Can you work these out from the model? Positions are in its coordinate system, mm. Face numbers are marked on the shaded views. Round coordinates to 2 decimals unless told otherwise and drop trailing zeros. Order: outer loops, then holes, each group sorted by start corner. A loop starts at its lowest first (then second) coordinate and runs counter-clockwise, first axis right, second up. Notation, with made-up numbers: M -38.75,31.25 L -34.75,31.25 A22 ccw -34.75,53.25 Z; hole C -12.5,59 d4. An arc over 180 degrees is marked long. Answer as a JSON object with one key per item and string values. Group by question number.
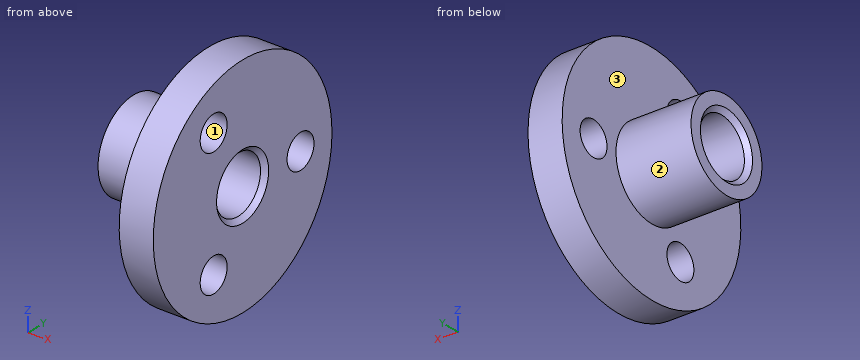
```python
from build123d import *

# Parameters (mm, degrees)
SKETCH_1_R               = 9.95
SKETCH_1_R_2             = 1.5
EXTRUDE_1_DEPTH          = 3
SKETCH_2_R               = 3.95
EXTRUDE_2_DEPTH          = 6.6
CUT_EXTRUDE_1_DEPTH      = 18.034230244
CUT_EXTRUDE_1_DEPTH_BACK = 18.034230244
SKETCH_3_R               = 2.5
CHAMFER_1_SIZE           = 0.4


with BuildPart() as part:
    # Эскиз1 → Бобышка-Вытянуть1 (new body)
    with BuildSketch(Plane(origin=(0, 0, 0), x_dir=(0, 0, -1), z_dir=(1, 0, 0))):
        Circle(SKETCH_1_R)
        with Locations((0, 6.45)):
            Circle(SKETCH_1_R_2, mode=Mode.SUBTRACT)
        with Locations((5.585863854, -3.225)):
            Circle(SKETCH_1_R_2, mode=Mode.SUBTRACT)
        with Locations((-5.585863854, -3.225)):
            Circle(SKETCH_1_R_2, mode=Mode.SUBTRACT)
    extrude(amount=EXTRUDE_1_DEPTH)

    # Эскиз2 → Бобышка-Вытянуть2 (add)
    with BuildSketch(Plane.ZY):
        with Locations(Location((0, 0, 0), (0, 0, 180))):
            Circle(SKETCH_2_R)
    extrude(amount=EXTRUDE_2_DEPTH)

    # Эскиз3 → Вырез-Вытянуть1 (cut, two sides: drawn at the far end of the back side and taken through both)
    with BuildSketch(Plane.ZY.offset(6.6).offset(-CUT_EXTRUDE_1_DEPTH_BACK)):
        Circle(SKETCH_3_R)
    extrude(amount=CUT_EXTRUDE_1_DEPTH + CUT_EXTRUDE_1_DEPTH_BACK, mode=Mode.SUBTRACT)

    # Фаска1
    chamfer_1_edges = [part.edges().sort_by_distance(p)[0] for p in [
        (-6.6, 0, -2.5),
        (3, 0, -2.5),
    ]]
    chamfer(chamfer_1_edges, length=CHAMFER_1_SIZE)


solid = part.part
```
1) For pin 1 (4 mm diameter, centred on y = -3.22, z = -5.59, fed in from +X); pin 2 (3 mm diameter, centred on x = -3.5, z = -1.5, fed in from -Y), each with a flat end and sliding along its axis, tell me the tip position at first contact or that it passes through.
2) If we section it at C-C on z = -4.5: Write out the boundary of the cut face in (x, y), plus the area to 3 significant figures.
3) If we section it at D-D on x = 0.75: Write out the boundary of the cut face in (y, z) (3 decimals), plus the area to 3 significant figures.
4) We'd pull the mould along Y, two halves only. Please class the marked faces 1, 2 and 3: +Y half, -Y half, draft (parallel to the pull), parting line (faces both ways), or undercut.
5) If we section it at A-A on y = 0: Write out the boundary of the cut face in (x, z).
6) If we section it at B-B on z = 0: Write out the boundary of the cut face in (x, y), plus the area to 3 significant figures.
7) I need wall thicknesses on line 1 along Y through (x, z) = (1.1, 0); line 2 along Y through (x, z) = (-0.5, 0); line 3 along X through (y, z) = (8.25, -2). Which ranges of each line are inside material? Lowest first, please.
Findings:
{
 "1": {"pin 1": "stops at x = 3", "pin 2": "stops at y = -3.95"},
 "2": {"outline": "M 0,-8.87 L 3,-8.87 L 3,-4.26 L 0,-4.26 Z; M 0,-2.19 L 3,-2.19 L 3,8.87 L 0,8.87 Z", "area": "47.0 mm^2"},
 "3": {"outline": "C 0,0 d19.9; hole C -3.225,-5.586 d3; hole C -3.225,5.586 d3; hole C 0,0 d5; hole C 6.45,0 d3", "area": "270 mm^2"},
 "4": {"face 1": "undercut", "face 2": "parting line", "face 3": "draft"},
 "5": {"outline": "M -6.6,-3.95 L 0,-3.95 L 0,-9.95 L 3,-9.95 L 3,-2.9 L 2.6,-2.5 L -6.2,-2.5 L -6.6,-2.9 Z; M -6.6,2.9 L -6.2,2.5 L 2.6,2.5 L 3,2.9 L 3,9.95 L 0,9.95 L 0,3.95 L -6.6,3.95 Z"},
 "6": {"outline": "M -6.6,-3.95 L 0,-3.95 L 0,-9.95 L 3,-9.95 L 3,-2.9 L 2.6,-2.5 L -6.2,-2.5 L -6.6,-2.9 Z; M -6.6,2.9 L -6.2,2.5 L 2.6,2.5 L 3,2.9 L 3,4.95 L 0,4.95 L 0,3.95 L -6.6,3.95 Z; M 0,7.95 L 3,7.95 L 3,9.95 L 0,9.95 Z", "area": "54.5 mm^2"},
 "7": {"line 1": "y = -9.95 to -2.5, 2.5 to 4.95, 7.95 to 9.95", "line 2": "y = -3.95 to -2.5, 2.5 to 3.95", "line 3": "x = 0 to 3"}
}
